Verification items for the finished model (mm, model axes). Give positions to 0.01 mm unless a question says otherwise; leave off trailing zeros. Write each loop counter-clockwise with the first axis right and the second up, starting at its lowest first coordinate (ties: lowest second). Pieces come first, ordered by that corner, then holes. Notation, with made-up numbers: M -13,-27 L 13,-27 A9 ccw 13,-19 Z; hole C 65,-2.5 d5. An arc over 180 degrees is marked long. Answer as a JSON object with one key per item and string values.
```python
from build123d import *

# Parameters (mm, degrees)
F0_W     = 110
F0_H     = 210
F1_DEPTH = 10
F2_R     = 4.99999


# Not quite as in the source:
# - a fillet or chamfer is up to 0.001 mm smaller than in the source, because OpenCascade refuses the exact size


with BuildPart() as f1:
    # F0 (on Top) → F1 (new body)
    with BuildSketch(Plane.XY):
        Rectangle(F0_W, F0_H)
    extrude(amount=F1_DEPTH)

    # F2 (radius 5 in the source; OpenCascade refuses exactly that, so slightly less here)
    f2_edges = [f1.edges().sort_by_distance(p)[0] for p in [
        (-55, 0, 10),
        (0, -105, 10),
        (0, -105, 0),
        (-55, -105, 5),
        (-55, 0, 0),
        (-55, 105, 5),
        (0, 105, 10),
        (0, 105, 0),
        (55, 105, 5),
        (55, 0, 10),
        (55, 0, 0),
        (55, -105, 5),
    ]]
    fillet(f2_edges, radius=F2_R)


solid = f1.part
```
1) Section check A-A on z = 2. Record the boundary of the cut face in (x, y).
Completed:
{"outline": "M -54,-100 A4 ccw -50,-104 L 50,-104 A4 ccw 54,-100 L 54,100 A4 ccw 50,104 L -50,104 A4 ccw -54,100 Z"}
2) Go/stop test with flat-tipped pins: pin 1 (1.5 mm diameter, centred on y = 83, z = 3, fed in from +X); pin 2 (1 mm diameter, centred on x = 42.5, z = 2, fed in from +Y); pin 3 (1.5 mm diameter, centred on y = 24, z = 1.5, fed in from +X). Record where each tip stops, or that it passes through.
Completed:
{"pin 1": "stops at x = 54.84", "pin 2": "stops at y = 104.33", "pin 3": "stops at x = 54.18"}
3) Thickness scan on L1, parallel to Y at x = -32, z = 5.5; L2, parallel to X at y = 9.5, z = 6.25; L3, parallel to X at y = -12, z = 4.5. Record the ranges inside material, lowest first.
Completed:
{"L1": "y = -104.97 to 104.97", "L2": "x = -54.84 to 54.84", "L3": "x = -54.97 to 54.97"}
